```python
from build123d import *

# Parameters (mm, degrees)
SKETCH8_R           = 7.5
BOSS_EXTRUDE1_DEPTH = 12


with BuildPart() as part:
    # Sketch8 → Boss-Extrude1 (new, symmetric)
    with BuildSketch(Plane.XY):
        Polygon((0, 0), (32, 0), (32, 25), (6, 25), (6, 7), (0, 7), align=None)
        with Locations((19, 13)):
            Circle(SKETCH8_R, mode=Mode.SUBTRACT)
    boss_extrude1 = extrude(amount=BOSS_EXTRUDE1_DEPTH, both=True)

    # Mirror1: Boss-Extrude1 across plane
    add(boss_extrude1.mirror(Plane(origin=(0, 0, 0), x_dir=(0, 0, 1), z_dir=(1, 0, 0))))


solid = part.part
```
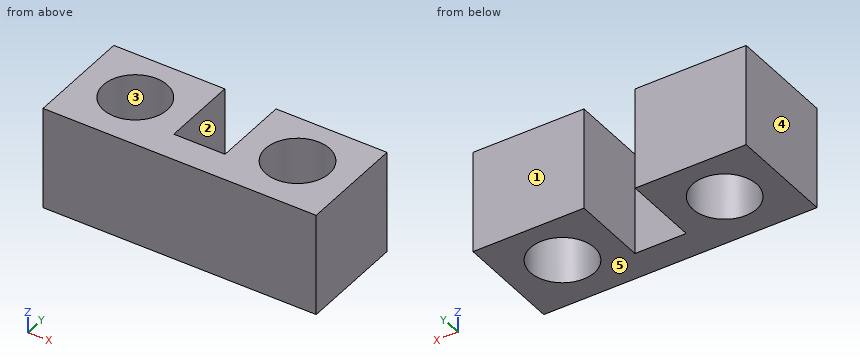
Verification items for the finished model (mm, model axes). Face numbers are marked on the shaded views. A direction names the side the tool comes from. Give positions to 0.01 mm unless a question says otherwise; leave off trailing zeros. Order: outer loops, then holes, each group sorted by start corner. A loop starts at its lowest first (then second) coordinate and runs counter-clockwise, first axis right, second up. Notation, with made-up numbers: (-37, -7.75) - (18, -7.75) arc R18 cw to (18, 20.25) - close; hole circle Ø8 at (23, -14). An arc over 180 degrees is marked (long way). Answer as CSV lines item,"result". Start each with the question number.
Item 1: Mould release check, pull along X, two halves, no side actions. Record for the marked faces 3, 4 and 5: released by +X, released by -X, zero draft, split by the parting line, or undercut.
Item 2: Access from +Z, -Z, +X, -X, +Y, -Y to the whole of each face (thin tool, end or side, straight path). Record for the marked faces 1 and 2.
Item 3: Section check C-C, the plane y = 13. Record the boundary of the cut face in (x, z), plus the area to 3 significant figures.
Item 4: Section check A-A, the plane z = -1.75. Record the boundary of the cut face in (x, y).
Item 5: Material ranges on L1, parallel to Y at x = 19, z = 6; L2, parallel to X at y = 7.5, z = -0.25; L3, parallel to X at y = 11.5, z = 4.25, recorded low to high.
Item 6: Section check D-D, the plane x = -20. Record the boundary of the cut face in (y, z).
Item 7: Gauge pin test, flat end, axial feed: pin 1 (13.5 mm diameter, centred on x = -19, y = 13, fed in from +Z). Record the tip position at first contact, or that the pin passes through.
Item 8: Section check B-B, the plane x = 19. Record the boundary of the cut face in (y, z).
Filled in:
1,face 3,"undercut"
1,face 4,"released by -X"
1,face 5,"zero draft"
2,face 1,"+Z, -Z, +X, -X, +Y"
2,face 2,"+Z, -Z, +Y"
3,outline,"(-32, -12) - (-26.5, -12) - (-26.5, 12) - (-32, 12) - close; (-11.5, -12) - (-6, -12) - (-6, 12) - (-11.5, 12) - close; (6, -12) - (11.5, -12) - (11.5, 12) - (6, 12) - close; (26.5, -12) - (32, -12) - (32, 12) - (26.5, 12) - close"
3,area,"528 mm^2"
4,outline,"(-32, 0) - (32, 0) - (32, 25) - (6, 25) - (6, 7) - (-6, 7) - (-6, 25) - (-32, 25) - close; hole circle Ø15 at (-19, 13); hole circle Ø15 at (19, 13)"
5,L1,"0 to 5.5, 20.5 to 25"
5,L2,"-32 to -24.1, -13.9 to -6, 6 to 13.9, 24.1 to 32"
5,L3,"-32 to -26.35, -11.65 to -6, 6 to 11.65, 26.35 to 32"
6,outline,"(0, -12) - (5.57, -12) - (5.57, 12) - (0, 12) - close; (20.43, -12) - (25, -12) - (25, 12) - (20.43, 12) - close"
7,pin 1,"through"
8,outline,"(0, -12) - (5.5, -12) - (5.5, 12) - (0, 12) - close; (20.5, -12) - (25, -12) - (25, 12) - (20.5, 12) - close"
